```python
from build123d import *

# Parameters (mm, degrees)
BOSS_EXTRUDE1_DEPTH = 12.7
SKETCH2_R           = 1.778
BOSS_EXTRUDE2_DEPTH = 6.35


with BuildPart() as part:
    # Sketch1 → Boss-Extrude1 (new body)
    with BuildSketch(Plane(origin=(0, 0, 0), x_dir=(1, 0, 0), z_dir=(0, 1, 0))):
        Polygon((0, 3.666174209), (-3.175, 1.833087105), (-3.175, -1.833087105), (0, -3.666174209), (3.175, -1.833087105), (3.175, 1.833087105), align=None)
    extrude(amount=BOSS_EXTRUDE1_DEPTH)

    # Sketch2 → Boss-Extrude2 (add)
    with BuildSketch(Plane(origin=(0, 12.7, 0), x_dir=(1, 0, 0), z_dir=(0, 1, 0))):
        Circle(SKETCH2_R)
    extrude(amount=BOSS_EXTRUDE2_DEPTH)


solid = part.part
```
Work out the finished part from the listing and answer in its coordinate system (mm). A direction names the side the tool comes from. Round coordinates to 2 decimals unless told otherwise and drop trailing zeros. Loops run counter-clockwise (first coordinate to the right, second up) from the corner with the lowest first, then second, coordinate; pieces in that order, holes last.
(1) The part is cut by section B-B, the plane y = 3. Give the vertices of the cut face in (x, z) (3 decimals).
Computed values:
outline: (-3.175, -1.833) - (0, -3.666) - (3.175, -1.833) - (3.175, 1.833) - (0, 3.666) - (-3.175, 1.833) - close
(2) The part is cut by section D-D, the plane y = 16.75. Give the vertices of the cut face in (x, z), and give its area (3 significant figures).
Computed values:
outline: circle Ø3.56 at (0, 0)
area: 9.93 mm2
(3) The part is cut by section A-A, the plane z = 0. Give the vertices of the cut face in (x, y) (3 decimals), and give its area (3 significant figures).
Computed values:
outline: (-3.175, 0) - (3.175, 0) - (3.175, 12.7) - (1.778, 12.7) - (1.778, 19.05) - (-1.778, 19.05) - (-1.778, 12.7) - (-3.175, 12.7) - close
area: 103 mm2
(4) Each of these flat-tipped pins is pushed along its axis until it touches: P1, Ø4, axis at y = 16, z = 1.5, coming from the +X side; P2, Ø3, axis at x = -2, y = 4.5, coming from the +Z side; P3, Ø3, axis at x = 1.5, z = -1, coming from the -Y side; P4, Ø2, axis at x = 0.5, y = 3, coming from the +Z side. Where does it stop, or does it pass through?
Computed values:
P1: stops at x = 1.78
P2: stops at z = 3.38
P3: stops at y = 0
P4: stops at z = 3.67
(5) Find the intervals of material crossed by L1, parallel to Y at x = 3, z = 0.75; L2, parallel to Z at x = 2.75, y = 12.5; L3, parallel to X at y = 5.75, z = -2, in increasing order.
Computed values:
L1: y = 0 to 12.7
L2: z = -2.08 to 2.08
L3: x = -2.89 to 2.89
(6) For faces 1 (the cylindrical face through (-0.385, 15.831, 1.736)), 2 (the flat face through (-3.175, 6, 0)), determine the directions among +Z, -Z, +X, -X, +Y, -Y from which every point of the face is accessible in a straight line to the end or side of a thin tool.
Computed values:
face 1: +Y
face 2: +Z, -Z, -X, +Y, -Y
(7) The part is cut by section C-C, the plane x = -0.5. Give the vertices of the cut face in (y, z), and give its area (3 significant figures).
Computed values:
outline: (0, -3.38) - (12.7, -3.38) - (12.7, -1.71) - (19.05, -1.71) - (19.05, 1.71) - (12.7, 1.71) - (12.7, 3.38) - (0, 3.38) - close
area: 107 mm2
